For this review, take the finished solid that the model builds, in its own axes (mm). A direction names the side the tool comes from. Coordinates: 2 decimals unless noted, no trailing zeros. Write each loop counter-clockwise with the first axis right and the second up, starting at its lowest first coordinate (ties: lowest second). Pieces come first, ordered by that corner, then holes. Notation, with made-up numbers: (88.5, 62) - (109.5, 62) arc R21 ccw to (109.5, 90) - close; hole circle Ø10 at (77.25, 81.5). An arc over 180 degrees is marked (long way). Write each question's results on one line, items separated by ' | '.
from build123d import *

# Parameters (mm, degrees)
SKETCH1_W           = 60.3
SKETCH1_H           = 34.5
SKETCH1_R           = 2
SKETCH1_W_2         = 40.3
SKETCH1_H_2         = 19.5
BOSS_EXTRUDE1_DEPTH = 7.46
SKETCH3_W           = 54
SKETCH3_H           = 19.5
CUT_EXTRUDE1_DEPTH  = 2.5
SKETCH4_R           = 2.5
CUT_EXTRUDE2_DEPTH  = 36.527969264


with BuildPart() as part:
    # Sketch1 → Boss-Extrude1 (new body)
    with BuildSketch(Plane(origin=(0, 0, 0), x_dir=(1, 0, 0), z_dir=(0, 1, 0))):
        Rectangle(SKETCH1_W, SKETCH1_H)
        with Locations(Location((-24.315, -5, 0), (0, 0, 90))):
            Circle(SKETCH1_R, mode=Mode.SUBTRACT)
        with Locations(Location((-24.315, 5, 0), (0, 0, 90))):
            Circle(SKETCH1_R, mode=Mode.SUBTRACT)
        with Locations(Location((24.315, -5, 0), (0, 0, 90))):
            Circle(SKETCH1_R, mode=Mode.SUBTRACT)
        with Locations(Location((24.315, 5, 0), (0, 0, 90))):
            Circle(SKETCH1_R, mode=Mode.SUBTRACT)
        Rectangle(SKETCH1_W_2, SKETCH1_H_2, mode=Mode.SUBTRACT)
    extrude(amount=BOSS_EXTRUDE1_DEPTH)

    # Sketch3 → Cut-Extrude1 (cut)
    with BuildSketch(Plane(origin=(0, 7.46, 0), x_dir=(1, 0, 0), z_dir=(0, 1, 0))):
        Rectangle(SKETCH3_W, SKETCH3_H)
    extrude(amount=-CUT_EXTRUDE1_DEPTH, mode=Mode.SUBTRACT)

    # Sketch4 → Cut-Extrude2 (cut, through all)
    with BuildSketch(Plane(origin=(0, 7.46, 0), x_dir=(1, 0, 0), z_dir=(0, 1, 0))):
        with Locations(Location((0, 13.5, 0), (0, 0, 270))):
            Circle(SKETCH4_R)
        with Locations(Location((8, 13.5, 0), (0, 0, 270))):
            Circle(SKETCH4_R)
        with Locations(Location((16, 13.5, 0), (0, 0, 270))):
            Circle(SKETCH4_R)
        with Locations(Location((24, 13.5, 0), (0, 0, 270))):
            Circle(SKETCH4_R)
        with Locations(Location((-24, 13.5, 0), (0, 0, 270))):
            Circle(SKETCH4_R)
        with Locations(Location((-16, 13.5, 0), (0, 0, 270))):
            Circle(SKETCH4_R)
        with Locations(Location((-8, 13.5, 0), (0, 0, 270))):
            Circle(SKETCH4_R)
        with Locations(Location((24, -13.5, 0), (0, 0, 270))):
            Circle(SKETCH4_R)
        with Locations(Location((16, -13.5, 0), (0, 0, 270))):
            Circle(SKETCH4_R)
        with Locations(Location((8, -13.5, 0), (0, 0, 270))):
            Circle(SKETCH4_R)
        with Locations(Location((0, -13.5, 0), (0, 0, 270))):
            Circle(SKETCH4_R)
        with Locations(Location((-8, -13.5, 0), (0, 0, 270))):
            Circle(SKETCH4_R)
        with Locations(Location((-16, -13.5, 0), (0, 0, 270))):
            Circle(SKETCH4_R)
        with Locations(Location((-24, -13.5, 0), (0, 0, 270))):
            Circle(SKETCH4_R)
    extrude(amount=-CUT_EXTRUDE2_DEPTH, mode=Mode.SUBTRACT)


solid = part.part
Q1. For pin 1 (8 mm diameter, centred on x = 16, z = -13.5, fed in from +Y); pin 2 (3 mm diameter, centred on x = -16, z = -13.5, fed in from +Y), all flat-tipped, find the tip position at first contact; note any pin that passes through.
Results found:
pin 1: y = 7.46 | pin 2: through
Q2. Take a section at A-A on z = 12. State how many separate pieces and enclosed holes the cut face has, plus the area to 3 significant figures.
Results found:
separate pieces: 8 | enclosed holes: 0 | area: 241 mm2
Q3. Take a section at C-C on x = 16. State the section outline as (y, z) points.
Results found:
outline: (0, -17.25) - (7.46, -17.25) - (7.46, -16) - (0, -16) - close; (0, -11) - (7.46, -11) - (7.46, -9.75) - (0, -9.75) - close; (0, 9.75) - (7.46, 9.75) - (7.46, 11) - (0, 11) - close; (0, 16) - (7.46, 16) - (7.46, 17.25) - (0, 17.25) - close
Q4. Mouldability with a two-part tool opening along X and no side actions: class faces 1 (the face through (22.96, 2.45, -3.53)), 2 (the face through (30.15, 4, 0)), 3 (the face through (0, 4, 17.25)) as pulls with the +X half, pulls with the -X half, needs draft (parallel to the pull), parting line crosses it, or undercut.
Results found:
face 1: undercut | face 2: pulls with the +X half | face 3: needs draft
Q5. Wall thickness on line 1 along X through (y, z) = (4.5, -5) (3 decimals); line 2 along Z through (x, y) = (20, 4); line 3 along Z through (x, y) = (-18, 0.75): over which ranges is each line inside the solid? List them lowest first. Write a range as from..to.
Results found:
line 1: -30.15..-26.315, -22.315..-20.15, 20.15..22.315, 26.315..30.15 | line 2: -17.25..-9.75, 9.75..17.25 | line 3: -17.25..-15, -12..-9.75, 9.75..12, 15..17.25
Q6. For faces 4 (the face through (-30.15, 4, 0)), 5 (the face through (-24, 4.96, 0)), 6 (the face through (20.15, 2, 0)), list the 3-axis set-ups (+Z, -Z, +X, -X, +Y, -Y) from which the entire face can be reached by the end or side of a thin tool; tool diameter is ignored.
Results found:
face 4: +Z, -Z, -X, +Y, -Y | face 5: +Y | face 6: +Y, -Y
Q7. Take a section at D-D on z = -1.5. State the section outline as (x, y) points, plus the area to 3 significant figures.
Results found:
outline: (-30.15, 0) - (-20.15, 0) - (-20.15, 4.96) - (-27, 4.96) - (-27, 7.46) - (-30.15, 7.46) - close; (20.15, 0) - (30.15, 0) - (30.15, 7.46) - (27, 7.46) - (27, 4.96) - (20.15, 4.96) - close | area: 115 mm2
